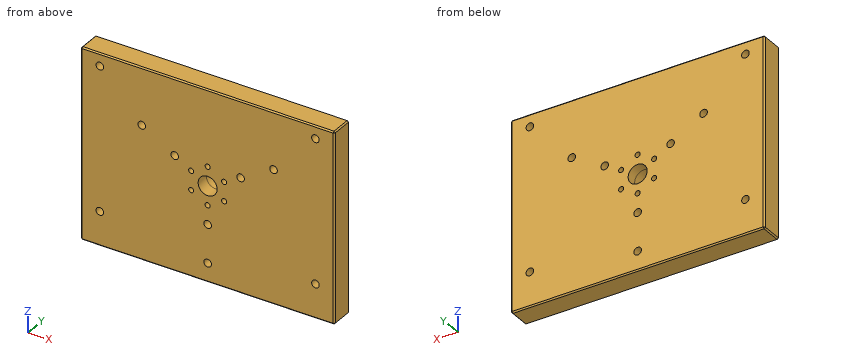
```python
from build123d import *

# Parameters (mm, degrees)
SKETCH1_W                = 200
SKETCH1_H                = 150
SKETCH1_R                = 7.5
SKETCH1_R_2              = 2
BOSS_EXTRUDE1_DEPTH      = 8
BOSS_EXTRUDE1_DEPTH_BACK = 10
SKETCH2_R                = 3
CUT_EXTRUDE2_DEPTH       = 10
CUT_EXTRUDE2_DEPTH_BACK  = 10
CHAMFER2_SIZE            = 1


with BuildPart() as part:
    # Sketch1 → Boss-Extrude1 (new body, two sides)
    with BuildSketch(Plane(origin=(0, 0, 0), x_dir=(1, 0, 0), z_dir=(0, 1, 0))) as boss_extrude1_sk:
        Rectangle(SKETCH1_W, SKETCH1_H)
        Circle(SKETCH1_R, mode=Mode.SUBTRACT)
        with Locations((0, 15)):
            Circle(SKETCH1_R_2, mode=Mode.SUBTRACT)
        with Locations((12.990381057, 7.5)):
            Circle(SKETCH1_R_2, mode=Mode.SUBTRACT)
        with Locations((12.990381057, -7.5)):
            Circle(SKETCH1_R_2, mode=Mode.SUBTRACT)
        with Locations((0, -15)):
            Circle(SKETCH1_R_2, mode=Mode.SUBTRACT)
        with Locations((-12.990381057, -7.5)):
            Circle(SKETCH1_R_2, mode=Mode.SUBTRACT)
        with Locations((-12.990381057, 7.5)):
            Circle(SKETCH1_R_2, mode=Mode.SUBTRACT)
    extrude(amount=BOSS_EXTRUDE1_DEPTH)
    extrude(boss_extrude1_sk.sketch, amount=-BOSS_EXTRUDE1_DEPTH_BACK)

    # Sketch2 → Cut-Extrude2 (cut, two sides)
    with BuildSketch(Plane(origin=(0, 0, 0), x_dir=(1, 0, 0), z_dir=(0, 1, 0))) as cut_extrude2_sk:
        with Locations((-25.980762114, -15)):
            Circle(SKETCH2_R)
        with Locations((0, 30)):
            Circle(SKETCH2_R)
        with Locations((25.980762114, -15)):
            Circle(SKETCH2_R)
        with Locations((85, 48)):
            Circle(SKETCH2_R)
        with Locations((85, -65)):
            Circle(SKETCH2_R)
        with Locations((-51.961524227, -30)):
            Circle(SKETCH2_R)
        with Locations((-85, -65)):
            Circle(SKETCH2_R)
        with Locations((-85, 48)):
            Circle(SKETCH2_R)
        with Locations((0, 60)):
            Circle(SKETCH2_R)
        with Locations((51.961524227, -30)):
            Circle(SKETCH2_R)
    extrude(amount=CUT_EXTRUDE2_DEPTH, mode=Mode.SUBTRACT)
    extrude(cut_extrude2_sk.sketch, amount=-CUT_EXTRUDE2_DEPTH_BACK, mode=Mode.SUBTRACT)

    # Chamfer2
    chamfer2_edges = [part.edges().sort_by_distance(p)[0] for p in [
        (-100, -10, 0),
        (0, -10, 75),
        (100, 8, 0),
        (0, 8, -75),
        (-100, 8, 0),
        (0, 8, 75),
        (100, -10, 0),
        (0, -10, -75),
        (100, -1, 75),
        (-100, -1, 75),
        (-100, -1, -75),
        (100, -1, -75),
    ]]
    chamfer(chamfer2_edges, length=CHAMFER2_SIZE)


solid = part.part
```
Work out the finished part from the listing and answer in its coordinate system (mm). Give positions to 0.01 mm unless a question says otherwise; leave off trailing zeros. Write each loop counter-clockwise with the first axis right and the second up, starting at its lowest first coordinate (ties: lowest second). Pieces come first, ordered by that corner, then holes.
(1) The part is cut by section A-A on x = 85. Write down the section's boundary in (y, z), plus the area to 3 significant figures.
Final values:
outline: (-10, -74) - (-9, -75) - (7, -75) - (8, -74) - (8, -51) - (-10, -51) - close; (-10, -45) - (8, -45) - (8, 62) - (-10, 62) - close; (-10, 68) - (8, 68) - (8, 74) - (7, 75) - (-9, 75) - (-10, 74) - close
area: 2,480 mm2
(2) Straight lines are drawn through the part: line 1 (Z direction, x = -85, y = 2); line 2 (X direction, y = 2.5, z = 30); line 3 (X direction, y = 5.75, z = 65). For each, find the intervals that lie inside material, in ascending order.
Final values:
line 1: z = -75 to -51, -45 to 62, 68 to 75
line 2: x = -100 to -54.96, -48.96 to 48.96, 54.96 to 100
line 3: x = -100 to -88, -82 to 82, 88 to 100
(3) The part is cut by section B-B on z = 65. Write down the section's boundary in (x, y).
Final values:
outline: (-100, -9) - (-99, -10) - (-88, -10) - (-88, 8) - (-99, 8) - (-100, 7) - close; (-82, -10) - (82, -10) - (82, 8) - (-82, 8) - close; (88, -10) - (99, -10) - (100, -9) - (100, 7) - (99, 8) - (88, 8) - close
(4) The part is cut by section C-C on y = -6.25. Count the separate pieces of the cut face and the enclosed holes in it, plus the area to 3 significant figures.
Final values:
separate pieces: 1
enclosed holes: 17
area: 29,500 mm2
(5) A flat-ended cylindrical pin translates along its axis: pin 1 Ø12 at (x, z) = (0, 0) entering from +Y. Find the tip coordinate at first contact, or state that the pin passes through.
Final values:
pin 1: passes through
